from build123d import *

# Parameters (mm, degrees)
F1_DEPTH = 3.175


with BuildPart() as f1:
    # F0 (on Top) → F1 (new body)
    with BuildSketch(Plane.XY):
        Polygon((-222.5, -40.4475), (222.5, -40.4475), (176.6197321826, 40.4475), (141.6947321826, 40.4475), (11.5447321826, 40.4475), (-23.3802678174, 40.4475), align=None)
        with BuildLine():
            ThreePointArc((-116.282366584, -16.3878218263), (-114.1217077206, -16.6117685547), (-113.1009845959, -18.5292468893))
            ThreePointArc((-113.1009845959, -18.5292468893), (-116.7030614712, -20.4467252239), (-116.282366584, -16.3878218263))
        make_face(mode=Mode.SUBTRACT)
        with BuildLine():
            ThreePointArc((11.5447321826, -4.2411), (13.1791387966, -4.918093386), (13.8561321826, -6.5525))
            ThreePointArc((13.8561321826, -6.5525), (9.9103255685, -8.186906614), (11.5447321826, -4.2411))
        make_face(mode=Mode.SUBTRACT)
        with BuildLine():
            ThreePointArc((141.6947321826, -4.2411), (143.3291387966, -4.918093386), (144.0061321826, -6.5525))
            ThreePointArc((144.0061321826, -6.5525), (140.0603255685, -8.186906614), (141.6947321826, -4.2411))
        make_face(mode=Mode.SUBTRACT)
        with BuildLine():
            ThreePointArc((184.1736370913, -8.7264269389), (184.3980129389, -9.2770651231), (184.4744918977, -9.8667242618))
            ThreePointArc((184.4744918977, -9.8667242618), (179.9281708566, -10.4563834005), (184.1736370913, -8.7264269389))
        make_face(mode=Mode.SUBTRACT)
    extrude(amount=F1_DEPTH)


solid = f1.part
Verification items for the finished model (mm, model axes). Round coordinates to 2 decimals unless told otherwise and drop trailing zeros. Order: outer loops, then holes, each group sorted by start corner. A loop starts at its lowest first (then second) coordinate and runs counter-clockwise, first axis right, second up.
1. Section check C-C on y = 24. Record the cut outline in (x, z) (3 decimals).
Final values:
outline: (-63.865, 0) - (185.948, 0) - (185.948, 3.175) - (-63.865, 3.175) - close
2. Section check A-A on z = 0.9. Record the cut outline in (x, y).
Final values:
outline: (-222.5, -40.45) - (222.5, -40.45) - (176.62, 40.45) - (-23.38, 40.45) - close; hole circle Ø4.62 at (-115.41, -18.53); hole circle Ø4.62 at (11.54, -6.55); hole circle Ø4.62 at (141.69, -6.55); hole circle Ø4.62 at (182.16, -9.87)
3. Section check B-B on x = -76. Record the cut outline in (y, z) (1 decimal), then the cut area to 3 significant figures.
Final values:
outline: (-40.4, 0) - (19.1, 0) - (19.1, 3.2) - (-40.4, 3.2) - close
area: 189 mm2
4. Thickness scan on L1, parallel to X at y = -8.5, z = 0.7; L2, parallel to X at y = -10.5, z = 0.5; L3, parallel to X at y = -20, z = 2.45. Record the ranges inside material, lowest first.
Final values:
L1: x = -143.86 to 10.3, 12.79 to 140.45, 142.94 to 180.3, 184.03 to 204.38
L2: x = -148.79 to 179.94, 184.39 to 205.52
L3: x = -172.17 to -117.2, -113.63 to 210.9
